Input: part model. Units: mm. Frame: model coordinates. Face numbers are marked on the shaded views. A direction names the side the tool comes from. Give positions to 0.01 mm unless a question says otherwise; leave off trailing zeros. Loops run counter-clockwise (first coordinate to the right, second up) from the corner with the lowest first, then second, coordinate; pieces in that order, holes last. Notation, with made-up numbers: M 30.5,12 L 87.5,12 A19 cw 87.5,16 Z; hole C -28.75,78.25 d4. An arc over 180 degrees is marked long. One line per item, written item: value. Start each with the question number.
(1) Section C-C on x = 21.5. Output: boundary loops of the cut face in (y, z).
(2) Ray query, line 1 along X through (y, z) = (-10, -34.25); line 2 along Y through (x, z) = (15, -33.25); line 3 along X through (y, z) = (6.5, -33). Return the intervals inside material, ascending. Write a range as from..to.
(3) Section A-A on y = 2. Output: boundary loops of the cut face in (x, z).
(4) Section B-B on y = -10. State how many separate pieces and enclosed holes the cut face has, plus the area to 3 significant figures.
(5) Pin query (flat end, axial travel): P1, Ø5, axis at x = -4, y = -5.5, coming from the +Z side; P2, Ø2.5, axis at x = 69.5, z = -33.5, coming from the +Y side; P3, Ø2.5, axis at x = 127.5, z = -26, coming from the -Y side; P4, Ø5, axis at y = 8.43, z = -27.89, coming from the -X side. Return the tip coordinate at first contact, or that it passes through.
(6) Access query for the marked faces 1 and 2. Directions: +Z, -Z, +X, -X, +Y, -Y. A direction counts if a zero-diameter tool reaches every point of the face in a straight line with its end or side. Return the directions, or none.
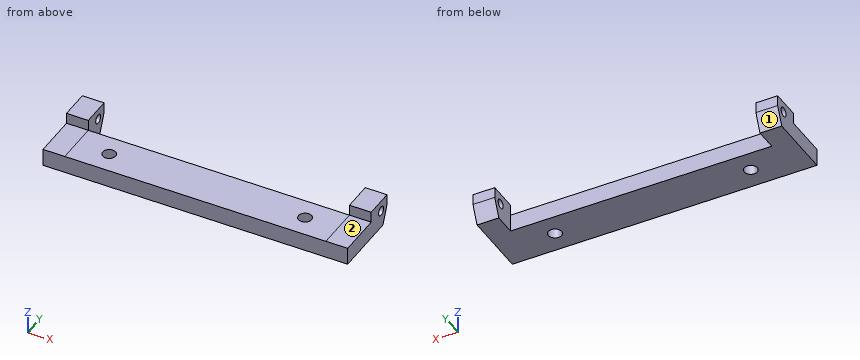
```python
from build123d import *

# Parameters (mm, degrees)
SKETCH_1_R          = 2.1
EXTRUDE_1_DEPTH     = 10
SKETCH_2_R          = 2.1
EXTRUDE_2_DEPTH     = 10
EXTRUDE_3_DEPTH     = 20
SKETCH_4_R          = 3
CUT_EXTRUDE_1_DEPTH = 20


with BuildPart() as part:
    # Sketch 1 → Extrude 1 (new body)
    with BuildSketch(Plane(origin=(120, 0, 0), x_dir=(0, 0, -1), z_dir=(1, 0, 0))):
        Polygon((27.888881523, 13.434002899), (36, 10), (36, -20), (27.958257708, -20), (27.958257708, 0), (22.958257708, 0), (22.958257708, 13.434002899), align=None)
        with Locations((27.888881523, 8.434002899)):
            Circle(SKETCH_1_R, mode=Mode.SUBTRACT)
    extrude(amount=EXTRUDE_1_DEPTH)



with BuildPart() as body_2:
    # Sketch 2 → Extrude 2 (new body)
    with BuildSketch(Plane.ZY):
        Polygon((-22.958257708, 13.434002899), (-27.888881523, 13.434002899), (-36, 10), (-36, -20), (-27.958257708, -20), (-27.958257708, 0), (-22.958257708, 0), align=None)
        with Locations(Location((-27.888881523, 8.434002899, 0), (0, 0, 180))):
            Circle(SKETCH_2_R, mode=Mode.SUBTRACT)
    extrude(amount=EXTRUDE_2_DEPTH)


with BuildPart() as part_1:
    add(part.part)

    add(body_2.part)  # Extrude 3 merges body 2
    # Sketch 3 → Extrude 3 (add)
    with BuildSketch(Plane(origin=(0, 0, 0), x_dir=(-1, 0, 0), z_dir=(0, -1, 0))):
        Polygon((-120, 27.975706714), (0, 27.958257708), (0, 36), (-120, 36), align=None)
    extrude(amount=EXTRUDE_3_DEPTH)

    # Sketch 4 → Cut-Extrude 1 (cut)
    with BuildSketch(Plane(origin=(-0.004065365, 0, -27.958257117), x_dir=(0.9999999894282007, 0, -0.00014540838614521652), z_dir=(0.00014540838614521652, 0, 0.9999999894282007))):
        with Locations((15.004065365, -10)):
            Circle(SKETCH_4_R)
        with Locations((105.004064097, -10)):
            Circle(SKETCH_4_R)
    extrude(amount=-CUT_EXTRUDE_1_DEPTH, mode=Mode.SUBTRACT)


solid = part_1.part
```
Output values:
1. outline: M -20,-36 L 0,-36 L 0,-27.96 L -20,-27.96 Z
2. line 1: x = -10..12, 18..102, 108..130
2. line 2: y = -20..-13, -7..0
2. line 3: x = -10..0, 120..130
3. outline: M -10,-36 L 0,-36 L 0,-22.96 L -10,-22.96 Z; M 120,-36 L 130,-36 L 130,-22.96 L 120,-22.96 Z
4. separate pieces: 3
4. enclosed holes: 0
4. area: 1,030 mm²
5. P1: stops at z = -27.96
5. P2: stops at y = 0
5. P3: stops at y = 0
5. P4: stops at x = -10
6. face 1: -Z, +X, -X, +Y
6. face 2: +Z, +X, -X, -Y
